Build history of the part. All positions in model axes, mm. A direction names the side the tool comes from. Give positions to 0.01 mm unless a question says otherwise; leave off trailing zeros. Write each loop counter-clockwise with the first axis right and the second up, starting at its lowest first coordinate (ties: lowest second). Pieces come first, ordered by that corner, then holes.
from build123d import *

# Parameters (mm, degrees)
SKETCH1_R            = 10.8
SKETCH1_R_2          = 9.8
BOSS_EXTRUDE7_DEPTH  = 35
SKETCH1_10_R         = 9.8
BOSS_EXTRUDE8_DEPTH  = 1
BOSS_EXTRUDE9_DEPTH  = 5
SKETCH1_13_W         = 2.9
SKETCH1_13_H         = 0.75
BOSS_EXTRUDE10_DEPTH = 2
BOSS_EXTRUDE11_DEPTH = 0.5
BOSS_EXTRUDE12_DEPTH = 20


with BuildPart() as part:
    # Sketch1 → Boss-Extrude7 (new body)
    with BuildSketch(Plane(origin=(0, 0, 0), x_dir=(1, 0, 0), z_dir=(0, 1, 0))):
        with Locations(Location((0, 0, 0), (0, 0, 270))):
            Circle(SKETCH1_R)
        with Locations(Location((0, 0, 0), (0, 0, 270))):
            Circle(SKETCH1_R_2, mode=Mode.SUBTRACT)
    extrude(amount=BOSS_EXTRUDE7_DEPTH)

    # Sketch1_10 → Boss-Extrude8 (add)
    with BuildSketch(Plane(origin=(0, 0, 0), x_dir=(1, 0, 0), z_dir=(0, 1, 0))):
        with Locations(Location((0, 0, 0), (0, 0, 270))):
            Circle(SKETCH1_10_R)
        Polygon((-2.35, 0), (-5.25, 0), (-7.25, 0), (-7.25, 3.75), (-5.25, 3.75), (5.25, 3.75), (7.25, 3.75), (7.25, 0), (5.25, 0), (2.35, 0), (2.35, -1), (-2.35, -1), align=None, mode=Mode.SUBTRACT)
    extrude(amount=BOSS_EXTRUDE8_DEPTH)

    # Sketch1_12 → Boss-Extrude9 (add)
    with BuildSketch(Plane(origin=(0, 0, 0), x_dir=(1, 0, 0), z_dir=(0, 1, 0))):
        Polygon((-5.25, 0), (-5.25, 0.75), (-6.5, 0.75), (-6.5, 3), (6.5, 3), (6.5, 0.75), (5.25, 0.75), (5.25, 0), (7.25, 0), (7.25, 3.75), (-7.25, 3.75), (-7.25, 0), align=None)
    extrude(amount=BOSS_EXTRUDE9_DEPTH)

    # Sketch1_13 → Boss-Extrude10 (add)
    with BuildSketch(Plane(origin=(0, 0, 0), x_dir=(1, 0, 0), z_dir=(0, 1, 0))):
        with Locations((-3.8, 0.375)):
            Rectangle(SKETCH1_13_W, SKETCH1_13_H)
        with Locations((3.8, 0.375)):
            Rectangle(SKETCH1_13_W, SKETCH1_13_H)
    extrude(amount=BOSS_EXTRUDE10_DEPTH)

    # Sketch1_14 → Boss-Extrude11 (add)
    with BuildSketch(Plane(origin=(0, 0, 0), x_dir=(1, 0, 0), z_dir=(0, 1, 0))):
        Polygon((-6.5, 0.75), (-5.25, 0.75), (-2.35, 0.75), (-2.35, 3), (-5.25, 3), (-6.5, 3), align=None)
        Polygon((5.25, 3), (2.35, 3), (2.35, 0.75), (5.25, 0.75), (6.5, 0.75), (6.5, 3), align=None)
    extrude(amount=BOSS_EXTRUDE11_DEPTH)

    # Sketch1_15 → Boss-Extrude12 (add)
    with BuildSketch(Plane(origin=(0, 0, 0), x_dir=(1, 0, 0), z_dir=(0, 1, 0))):
        Polygon((-5.25, 0), (-5.25, 0.75), (-6.5, 0.75), (-6.5, 3), (-5.25, 3), (-5.25, 3.75), (-7.25, 3.75), (-7.25, 0), align=None)
        Polygon((5.25, 3.75), (5.25, 3), (6.5, 3), (6.5, 0.75), (5.25, 0.75), (5.25, 0), (7.25, 0), (7.25, 3.75), align=None)
    extrude(amount=BOSS_EXTRUDE12_DEPTH)


solid = part.part
1. Mould opens along Z. For faces 1 (the face through (0, 3, -3)), 2 (the face through (0, 0, 2)), 3 (the face through (3.244, 17.255, 10.301)), 4 (the face through (-7.25, 10, -2)) say: pulls with the +Z half, pulls with the -Z half, needs draft (parallel to the pull), parting line crosses it, or undercut.
2. Saw through at B-B on x = 0. Give the cut face in (y, z).
3. 3-axis set-ups, long thin cutter, end or side, ignore diameter. For faces 5 (the face through (6, 10, 0)), 6 (the face through (0, 0.5, 1)), 7 (the face through (-10, 35, 2)): which of +Z, -Z, +X, -X, +Y, -Y reach the whole face in a straight line?
4. Drop flat-ended pins along their axis: pin 1 (2 mm diameter, centred on x = 6.5, z = -1, fed in from +Y); pin 2 (0.7 mm diameter, centred on x = -4.5, z = -1.5, fed in from +Y); pin 3 (2 mm diameter, centred on x = -5, y = 9.5, fed in from -Z). Give the stop position or say it passes through.
5. Saw through at A-A on y = 16.5. Give the cut face in (x, z), plus the area to 3 significant figures.
6. Saw through at D-D on y = 28.5. Give the cut face in (x, z), plus the area to 3 significant figures.
7. Saw through at C-C on z = -2. Give the cut face in (x, y).
8. Drill centre lines: line 1 along X through (y, z) = (22.5, 0); line 2 along Z through (x, y) = (-6.25, 18); line 3 along Z through (x, y) = (6, 17). Where is each one in solid material? Low to high.
Outcome:
1. face 1: undercut
1. face 2: needs draft
1. face 3: parting line crosses it
1. face 4: undercut
2. outline: (0, -10.8) - (35, -10.8) - (35, -9.8) - (1, -9.8) - (1, -3.75) - (5, -3.75) - (5, -3) - (0, -3) - close; (0, 1) - (1, 1) - (1, 9.8) - (35, 9.8) - (35, 10.8) - (0, 10.8) - close
3. face 5: +Y
3. face 6: +Y, -Y
3. face 7: +Z, -Z, +X, -X, +Y
4. pin 1: stops at y = 20
4. pin 2: stops at y = 0.5
4. pin 3: stops at z = -10.03
5. outline: circle Ø21.6 at (0, 0); (-7.25, -3.75) - (-5.25, -3.75) - (-5.25, -3) - (-6.5, -3) - (-6.5, -0.75) - (-5.25, -0.75) - (-5.25, 0) - (-7.25, 0) - close; (5.25, -3.75) - (7.25, -3.75) - (7.25, 0) - (5.25, 0) - (5.25, -0.75) - (6.5, -0.75) - (6.5, -3) - (5.25, -3) - close; hole circle Ø19.6 at (0, 0)
5. area: 74.1 mm2
6. outline: circle Ø21.6 at (0, 0); hole circle Ø19.6 at (0, 0)
6. area: 64.7 mm2
7. outline: (-10.61, 0) - (-2.35, 0) - (-2.35, 0.5) - (-6.5, 0.5) - (-6.5, 20) - (-7.25, 20) - (-7.25, 1) - (-9.59, 1) - (-9.59, 35) - (-10.61, 35) - close; (2.35, 0) - (10.61, 0) - (10.61, 35) - (9.59, 35) - (9.59, 1) - (7.25, 1) - (7.25, 20) - (6.5, 20) - (6.5, 0.5) - (2.35, 0.5) - close
8. line 1: x = -10.8 to -9.8, 9.8 to 10.8
8. line 2: z = -8.81 to -7.55, -3.75 to -3, -0.75 to 0, 7.55 to 8.81
8. line 3: z = -8.98 to -7.75, -3.75 to -3, -0.75 to 0, 7.75 to 8.98
